Source: CAD feature listing. Evaluate the final solid. Frame: model axes, mm. Face numbers are marked on the shaded views. A direction names the side the tool comes from. Round coordinates to 2 decimals unless told otherwise and drop trailing zeros. Write each loop counter-clockwise with the first axis right and the second up, starting at its lowest first coordinate (ties: lowest second). Pieces come first, ordered by that corner, then holes.
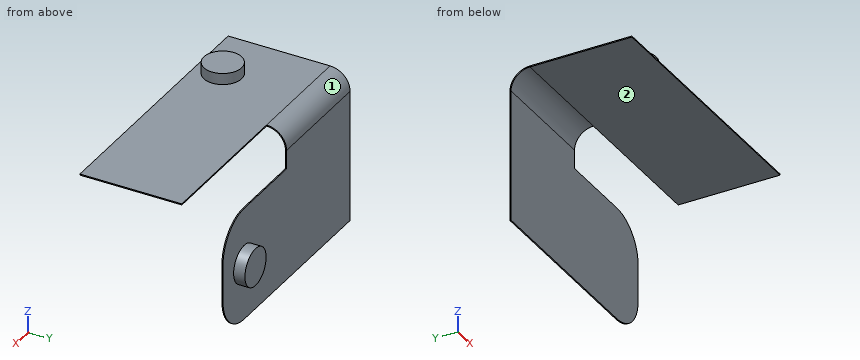
from build123d import *

# Parameters (mm, degrees)
SKETCH1_W           = 60
SKETCH1_H           = 30
BOSS_EXTRUDE1_DEPTH = 0.3
BOSS_EXTRUDE3_DEPTH = 30
SKETCH7_R           = 5
BOSS_EXTRUDE4_DEPTH = 3
SKETCH8_R           = 5
BOSS_EXTRUDE5_DEPTH = 3
SKETCH9_W           = 0.3
SKETCH9_H           = 27
BOSS_EXTRUDE6_DEPTH = 40
FILLET1_R           = 10


with BuildPart() as part:
    # Sketch1 → Boss-Extrude1 (new body)
    with BuildSketch(Plane(origin=(0, 0, 0), x_dir=(1, 0, 0), z_dir=(0, 1, 0))):
        with Locations((-33.606331541, -13.845258597)):
            Rectangle(SKETCH1_W, SKETCH1_H)
    extrude(amount=BOSS_EXTRUDE1_DEPTH)

    # Sketch6 → Boss-Extrude3 (add)
    with BuildSketch(Plane.ZY.offset(63.606331541)):
        with BuildLine():
            Line((28.845258597, 0.3), (33.845258597, 0.3))
            ThreePointArc((33.845258597, 0.3), (37.592924537, -1.25233406), (39.145258597, -5))
            Line((39.145258597, -5), (39.145258597, -32))
            Line((39.145258597, -32), (38.845258597, -32))
            Line((38.845258597, -32), (38.845258597, -5))
            ThreePointArc((38.845258597, -5), (37.380792503, -1.464466094), (33.845258597, 0))
            Line((33.845258597, 0), (28.845258597, 0))
            Line((28.845258597, 0), (28.845258597, 0.3))
        make_face()
    extrude(amount=-BOSS_EXTRUDE3_DEPTH)

    # Sketch7 → Boss-Extrude4 (add)
    with BuildSketch(Plane.XY.offset(39.145258597)):
        with Locations((-48.606331541, -25)):
            Circle(SKETCH7_R)
    extrude(amount=BOSS_EXTRUDE4_DEPTH)

    # Sketch8 → Boss-Extrude5 (add)
    with BuildSketch(Plane(origin=(0, 0.3, 0), x_dir=(1, 0, 0), z_dir=(0, 1, 0))):
        with Locations((-13.606331541, -13.845258597)):
            Circle(SKETCH8_R)
    extrude(amount=BOSS_EXTRUDE5_DEPTH)

    # Sketch9 → Boss-Extrude6 (add)
    with BuildSketch(Plane(origin=(-33.606331541, 0, 0), x_dir=(0, 0, -1), z_dir=(1, 0, 0))):
        with Locations((-38.995258597, -18.5)):
            Rectangle(SKETCH9_W, SKETCH9_H)
    extrude(amount=BOSS_EXTRUDE6_DEPTH)

    # Fillet1
    fillet1_edges = [part.edges().sort_by_distance(p)[0] for p in [
        (-3.606331541, 0.15, 28.845258597),
        (-3.606331541, 0.15, -1.154741403),
    ]]
    fillet(fillet1_edges, radius=FILLET1_R)


solid = part.part
1) Section query D-D on z = 23. Return the cut outline in (x, y).
Taken from the geometry:
outline: (-63.61, 0) - (-4.51, 0) - (-4.51, 0.3) - (-63.61, 0.3) - close
2) Section query B-B on y = -25. Return the cut outline in (x, z), then the cut area to 3 significant figures.
Taken from the geometry:
outline: (-63.61, 38.85) - (6.39, 38.85) - (6.39, 39.15) - (-43.61, 39.15) - (-43.61, 42.15) - (-53.61, 42.15) - (-53.61, 39.15) - (-63.61, 39.15) - close
area: 51.0 mm2
3) Section query A-A on x = -10. Return the cut outline in (y, z), then the cut area to 3 significant figures.
Taken from the geometry:
outline: (-32, 38.85) - (-5, 38.85) - (-5, 39.15) - (-32, 39.15) - close; (0, -0.48) - (0.3, -0.48) - (0.3, 10.38) - (3.3, 10.38) - (3.3, 17.31) - (0.3, 17.31) - (0.3, 28.17) - (0, 28.17) - close
area: 37.5 mm2
4) Reachability of the marked faces 1 and 2 from +Z, -Z, +X, -X, +Y, -Y: full face, straight path, thin tool, end or side. Return the list, or none.
Taken from the geometry:
face 1: +Z, +X, -X, +Y
face 2: -Z, +X, -X, -Y
5) Section query C-C on x = -40.5. Return the cut outline in (y, z), then the cut area to 3 significant figures.
Taken from the geometry:
outline: (-32, 38.85) - (-5, 38.85) arc R5 cw to (0, 33.85) - (0, -1.15) - (0.3, -1.15) - (0.3, 33.85) arc R5.3 ccw to (-5, 39.15) - (-32, 39.15) - close
area: 21.0 mm2
6) Contact query for flat-ended pins moving along their axis: P1, Ø6, axis at x = -36, z = 17.5, coming from the -Y side; P2, Ø8, axis at x = -37, z = 17.5, coming from the +Y side; P3, Ø4, axis at y = -2, z = 35.5, coming from the +X side. Output: stop coordinate, or through.
Taken from the geometry:
P1: stops at y = 0
P2: stops at y = 0.3
P3: stops at x = -33.61
7) Material intervals for line 1 (Y direction, x = -6.5, z = 18.5); line 2 (Y direction, x = -17, z = 17); line 3 (Z direction, x = -54, y = -8), sorted ascending.
Taken from the geometry:
line 1: y = 0 to 0.3
line 2: y = 0 to 3.3
line 3: z = 38.85 to 39.15
